from build123d import *

# Parameters (mm, degrees)
F1_DEPTH = 30.734
F2_DEPTH = 12.7
F3_R     = 6.6708512145
F4_DEPTH = 45.212
F5_DEPTH = 29.972


# Not quite as in the source:
# - a feature names something its author has since deleted; it is built from what else it names


with BuildPart() as f1:
    # F0 (on Right) → F1 (new body)
    with BuildSketch(Plane.YZ):
        Polygon((-28.4980535507, 0), (31.8277217448, 0), (31.8277217448, 37.6056805253), (9.8910769448, 37.6056805253), align=None)
    extrude(amount=F1_DEPTH)

    # F0 (on Right) → F2 (join)
    with BuildSketch(Plane.YZ):
        Polygon((-28.4980535507, 0), (31.8277217448, 0), (31.8277217448, 37.6056805253), (9.8910769448, 37.6056805253), align=None)
        Polygon((9.8910769448, 37.6056805253), (31.8277217448, 37.6056805253), (31.8277217448, 45.440196991), (9.8910769448, 45.440196991), (-36.4957887537, 0), (-28.4980535507, 0), align=None)
    extrude(amount=-F2_DEPTH)

    # F3 (on Front) → F4 (cut)
    with BuildSketch(Plane.XZ):
        with Locations((12.4372942373, 20.3697439283)):
            Circle(F3_R)
    extrude(amount=-F4_DEPTH, mode=Mode.SUBTRACT)

    # F3 (on Front) → F5 (cut)
    with BuildSketch(Plane.XZ):
        with Locations((12.4372942373, 20.3697439283)):
            Circle(F3_R)
    extrude(amount=F5_DEPTH, mode=Mode.SUBTRACT)


solid = f1.part
The listing builds one solid part. Answer for the finished solid, in the listing's coordinates (mm). A direction names the side the tool comes from. Give positions to 0.01 mm unless a question says otherwise; leave off trailing zeros. Write each loop counter-clockwise with the first axis right and the second up, starting at its lowest first coordinate (ties: lowest second). Pieces come first, ordered by that corner, then holes.
Item 1: Section B-B, the plane y = 5.5 is taken. Write down the section's boundary in (x, z).
Item 2: Which of the six approach directions +Z, -Z, +X, -X, +Y, -Y give full straight-line access (tool end or side, diameter ignored) to faces 1 (the flat face through (4, 31.828, 22)), 2 (the flat face through (15, 21, 37.606)), 3 (the flat face through (0, 0, 30))?
Item 3: Determine the mould class of faces 4 (the cylindrical face through (10.991, 13.482, 13.858)), 5 (the flat face through (30.734, 8, 15)), 6 (the flat face through (-6.261, -12.978, 23.038)) for opening direction X: released by +X, released by -X, zero draft, split by the parting line, or undercut.
Item 4: Section C-C, the plane x = -4 is taken. Write down the section's boundary in (y, z), plus the area to 3 significant figures.
Item 5: Flat-ended cylindrical pins translate along their axes: P1, Ø10.5, axis at x = 12.44, z = 20.37, coming from the -Y side; P2, Ø1.5, axis at x = 25, y = -18.5, coming from the +Z side; P3, Ø12, axis at x = 21.5, y = 15, coming from the +Z side; P4, Ø6, axis at x = 2.5, z = 11.5, coming from the -Y side. Find the tip coordinate at first contact, or state that the pin passes through.
Item 6: Section D-D, the plane z = 15.5 is taken. Write down the section's boundary in (x, y).
Item 7: Find the intervals of material crossed by line 1 along X through (y, z) = (-18.5, 16.5); line 2 along Z through (x, y) = (13, 15); line 3 along Z through (x, y) = (11, 19), in increasing order.
Item 8: Section A-A, the plane z = 23.5 is taken. Write down the section's boundary in (x, y).
Completed:
1. outline: (-12.7, 0) - (30.73, 0) - (30.73, 33.3) - (0, 33.3) - (0, 41.14) - (-12.7, 41.14) - close; hole circle Ø13.34 at (12.44, 20.37)
2. face 1: +Z, -Z, +X, -X, +Y
2. face 2: +Z, +X, +Y, -Y
2. face 3: +Z, +X, -Y
3. face 4: undercut
3. face 5: released by +X
3. face 6: zero draft
4. outline: (-36.5, 0) - (31.83, 0) - (31.83, 45.44) - (9.89, 45.44) - close
4. area: 2,050 mm2
5. P1: passes through
5. P2: stops at z = 10.53
5. P3: stops at z = 37.61
5. P4: stops at y = -26.45
6. outline: (-12.7, -20.67) - (0, -20.67) - (0, -12.68) - (7.88, -12.68) - (7.88, 31.83) - (-12.7, 31.83) - close; (17, -12.68) - (30.73, -12.68) - (30.73, 31.83) - (17, 31.83) - close
7. line 1: x = -12.7 to 0
7. line 2: z = 0 to 13.72, 27.02 to 37.61
7. line 3: z = 0 to 13.86, 26.88 to 37.61
8. outline: (-12.7, -12.51) - (0, -12.51) - (0, -4.51) - (6.55, -4.51) - (6.55, 31.83) - (-12.7, 31.83) - close; (18.33, -4.51) - (30.73, -4.51) - (30.73, 31.83) - (18.33, 31.83) - close
